Work out the finished part from the listing and answer in its coordinate system (mm). Face numbers are marked on the shaded views. Coordinates: 2 decimals unless noted, no trailing zeros. Order: outer loops, then holes, each group sorted by start corner. A loop starts at its lowest first (then second) coordinate and runs counter-clockwise, first axis right, second up. Notation, with made-up numbers: M 86,-18.5 L 128,-18.5 A24 ccw 128,16.5 Z; hole C 73.5,83.25 d9. An arc over 180 degrees is marked long. Write item = value, one per line. Start each with the question number.
Q1. Find section C-C on y = 12. Give the vertices of the cut face in (x, z), and give its area (3 significant figures).
Q2. Each of these flat-tipped pins is pushed along its axis until it touches: P1, Ø4.5, axis at x = 0, y = 24.3, coming from the +Z side; P2, Ø0.6, axis at x = 14, y = 1, coming from the -Z side (3 decimals); P3, Ø16, axis at x = 0, z = 0, coming from the +Y side. Where does it stop, or does it pass through?
Q3. Straight lines are drawn through the part: line 1 along Y through (x, z) = (0, -19); line 2 along X through (y, z) = (0.7, 0) (3 decimals); line 3 along X through (y, z) = (0.55, -16.55). For each, find the intervals that lie inside material, in ascending order.
Q4. Determine the mould class of the marked faces 1, 2 and 3 for opening direction Z: released by +Z, released by -Z, zero draft, split by the parting line, or undercut.
Q5. Find section D-D on z = -6. Give the vertices of the cut face in (x, y), and give its area (3 significant figures).
Q6. Find section B-B on x = -16. Give the vertices of the cut face in (y, z) (1 decimal).
Q7. Find section A-A on z = -16.55. Give the vertices of the cut face in (x, y), and give its area (3 significant figures).
```python
from build123d import *

# Parameters (mm, degrees)
ESQUISSE1_R        = 5
ESQUISSE1_R_2      = 1.6
BOSS_EXTRU_1_DEPTH = 2
ESQUISSE2_R        = 1.7
BOSS_EXTRU_2_DEPTH = 2
CONG_2_R           = 2
CONG_3_R           = 0.5


with BuildPart() as part:
    # Esquisse1 → Boss.-Extru.1 (new body)
    with BuildSketch(Plane(origin=(0, 0, 0), x_dir=(1, 0, 0), z_dir=(0, 1, 0))):
        with BuildLine():
            Line((-16.55, 3.625), (-12.5, 3.625))
            ThreePointArc((-12.5, 3.625), (-8.257359313, 5.382359313), (-6.5, 9.625))
            Line((-6.5, 9.625), (-6.5, 18.9))
            Line((-6.5, 18.9), (6.5, 18.9))
            Line((6.5, 18.9), (6.5, 9.625))
            ThreePointArc((6.5, 9.625), (8.257359313, 5.382359313), (12.5, 3.625))
            Line((12.5, 3.625), (16.55, 3.625))
            ThreePointArc((16.55, 3.625), (20.175, 0), (16.55, -3.625))
            Line((16.55, -3.625), (9.625, -3.625))
            ThreePointArc((9.625, -3.625), (5.382359313, -5.382359313), (3.625, -9.625))
            Line((3.625, -9.625), (3.625, -16.55))
            ThreePointArc((3.625, -16.55), (0, -20.175), (-3.625, -16.55))
            Line((-3.625, -16.55), (-3.625, -9.625))
            ThreePointArc((-3.625, -9.625), (-5.382359313, -5.382359313), (-9.625, -3.625))
            Line((-9.625, -3.625), (-16.55, -3.625))
            ThreePointArc((-16.55, -3.625), (-20.175, 0), (-16.55, 3.625))
        make_face()
        with Locations(Location((0, 0, 0), (0, 0, 270))):
            Circle(ESQUISSE1_R, mode=Mode.SUBTRACT)
        with Locations(Location((-9.55, 0, 0), (0, 0, 270))):
            Circle(ESQUISSE1_R_2, mode=Mode.SUBTRACT)
        with Locations(Location((-16.55, 0, 0), (0, 0, 270))):
            Circle(ESQUISSE1_R_2, mode=Mode.SUBTRACT)
        with Locations(Location((9.55, 0, 0), (0, 0, 90))):
            Circle(ESQUISSE1_R_2, mode=Mode.SUBTRACT)
        with Locations(Location((16.55, 0, 0), (0, 0, 90))):
            Circle(ESQUISSE1_R_2, mode=Mode.SUBTRACT)
        with Locations(Location((0, -9.55, 0), (0, 0, 90))):
            Circle(ESQUISSE1_R_2, mode=Mode.SUBTRACT)
        with Locations(Location((0, -16.55, 0), (0, 0, 90))):
            Circle(ESQUISSE1_R_2, mode=Mode.SUBTRACT)
        with Locations(Location((0, 16.55, 0), (0, 0, 270))):
            Circle(ESQUISSE1_R_2, mode=Mode.SUBTRACT)
        with Locations(Location((0, 9.55, 0), (0, 0, 270))):
            Circle(ESQUISSE1_R_2, mode=Mode.SUBTRACT)
    extrude(amount=BOSS_EXTRU_1_DEPTH)

    # Esquisse2 → Boss.-Extru.2 (add)
    with BuildSketch(Plane(origin=(0, 0, -18.9), x_dir=(-1, 0, 0), z_dir=(0, 0, -1))):
        with BuildLine():
            Line((-6.5, 0), (6.5, 0))
            Line((6.5, 0), (6.5, 2))
            Line((6.5, 2), (4.429285714, 24.3))
            ThreePointArc((4.429285714, 24.3), (0, 28.729285714), (-4.429285714, 24.3))
            Line((-4.429285714, 24.3), (-6.5, 2))
            Line((-6.5, 2), (-6.5, 0))
        make_face()
        with Locations((0, 24.3)):
            Circle(ESQUISSE2_R, mode=Mode.SUBTRACT)
        with Locations((0, 5.9)):
            Circle(ESQUISSE2_R, mode=Mode.SUBTRACT)
    extrude(amount=BOSS_EXTRU_2_DEPTH)

    # Congé2
    cong_2_edges = [part.edges().sort_by_distance(p)[0] for p in [
        (0, 0, -20.9),
    ]]
    fillet(cong_2_edges, radius=CONG_2_R)

    # Congé3
    cong_3_edges = [part.edges().sort_by_distance(p)[0] for p in [
        (0, 2, -18.9),
    ]]
    fillet(cong_3_edges, radius=CONG_3_R)


solid = part.part
```
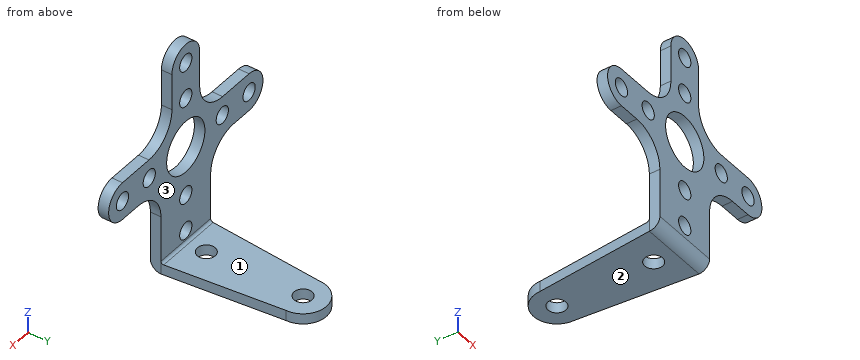
Findings below:
q1.outline = M -5.57,-20.9 L 5.57,-20.9 L 5.57,-18.9 L -5.57,-18.9 Z
q1.area = 22.3 mm^2
q2.P1 = -18.9
q2.P2 = -3.625
q2.P3 = 2
q3.line_1 = 0 to 4.2, 7.6 to 22.6, 26 to 28.73
q3.line_2 = -20.175 to -18.15, -14.95 to -11.15, -7.95 to -5, 5 to 7.95, 11.15 to 14.95, 18.15 to 20.175
q3.line_3 = -6.5 to -1.6, 1.6 to 6.5
q4.face_1 = released by +Z
q4.face_2 = released by -Z
q4.face_3 = zero draft
q5.outline = M -7.72,0 L 7.72,0 L 7.72,2 L -7.72,2 Z
q5.area = 30.9 mm^2
q6.outline = M 0,-3.6 L 2,-3.6 L 2,-1.5 L 0,-1.5 Z; M 0,1.5 L 2,1.5 L 2,3.6 L 0,3.6 Z
q7.outline = M -6.5,0 L -1.6,0 L -1.6,2 L -6.5,2 Z; M 1.6,0 L 6.5,0 L 6.5,2 L 1.6,2 Z
q7.area = 19.6 mm^2
